Read the model definition and answer for the solid it produces. Units are mm, in the model's axes. Face numbers are marked on the shaded views. Coordinates: 2 decimals unless noted, no trailing zeros. Write each loop counter-clockwise with the first axis right and the second up, starting at its lowest first coordinate (ties: lowest second). Pieces come first, ordered by that corner, then holes.
Item 1: Determine the mould class of the marked faces 1, 2 and 3 for opening direction Y: released by +Y, released by -Y, zero draft, split by the parting line, or undercut.
Item 2: Section B-B (z = 32.5) is taken. Give the vertices of the cut face in (x, y).
Item 3: Section D-D (z = 272) is taken. Give the vertices of the cut face in (x, y).
Item 4: Straight lines are drawn through the part: probe 1 along Y at (x, z) = (0, 131); probe 2 along X at (y, z) = (37.5, 284); probe 3 along Y at (x, z) = (17, 358). For each, find the intervals that lie inside material, in ascending order.
Item 5: Each of these flat-tipped pins is pushed along its axis until it touches: P1, Ø10, axis at x = -25, z = 162.5, coming from the +Y side; P2, Ø3, axis at x = -23, y = -11.5, coming from the +Z side; P3, Ø1.5, axis at x = -36, y = -36.5, coming from the -Z side. Where does it stop, or does it pass through?
Item 6: Section A-A (x = 0) is taken. Give the vertices of the cut face in (y, z), then the cut area to 3 significant figures.
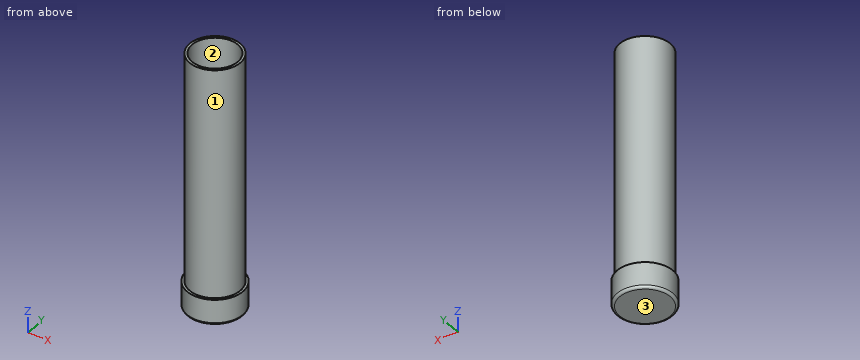
from build123d import *


with BuildPart() as f1:
    # F0 (on Front) → F1 (revolve)
    with BuildSketch(Plane.XZ):
        with BuildLine():
            ThreePointArc((-55, 5), (-53.535534, 1.464466), (-50, 0))
            Line((-50, 0), (-50, 50))
            Line((-50, 50), (-55, 50))
            Line((-55, 50), (-55, 5))
        make_face()
        Polygon((-50, 0), (0, 0), (0, 5), (-45, 5), (-45, 500), (-50, 500), (-50, 50), align=None)
    revolve(axis=Axis((0, 0, 252.5), (0, 0, -1)))


solid = f1.part
Established:
1. face 1: split by the parting line
1. face 2: undercut
1. face 3: zero draft
2. outline: circle Ø110 at (0, 0); hole circle Ø90 at (0, 0)
3. outline: circle Ø100 at (0, 0); hole circle Ø90 at (0, 0)
4. probe 1: y = -50 to -45, 45 to 50
4. probe 2: x = -33.07 to -24.87, 24.87 to 33.07
4. probe 3: y = -47.02 to -41.67, 41.67 to 47.02
5. P1: stops at y = 45.83
5. P2: stops at z = 5
5. P3: stops at z = 0.03
6. outline: (-55, 5) arc R5 ccw to (-50, 0) - (50, 0) arc R5 ccw to (55, 5) - (55, 50) - (50, 50) - (50, 500) - (45, 500) - (45, 5) - (-45, 5) - (-45, 500) - (-50, 500) - (-50, 50) - (-55, 50) - close
6. area: 5,940 mm2
